Read the model definition and answer for the solid it produces. Units are mm, in the model's axes. Give positions to 0.01 mm unless a question says otherwise; leave off trailing zeros. Use a Markdown table: item, result.
from build123d import *

# Parameters (mm, degrees)
SKETCH1_W           = 79.799999912
SKETCH1_H           = 81.28
BOSS_EXTRUDE1_DEPTH = 1.600000102
SKETCH2_R           = 1.524
CUT_EXTRUDE1_DEPTH  = 107.841239355
SKETCH4_R           = 1.6
CUT_EXTRUDE2_DEPTH  = 107.841239355


with BuildPart() as part:
    # Sketch1 → Boss-Extrude1 (new body)
    with BuildSketch(Plane(origin=(0, 0, 0), x_dir=(1, 0, 0), z_dir=(0, 1, 0))):
        with Locations((-31.957523467, -38.410532915)):
            Rectangle(SKETCH1_W, SKETCH1_H)
    extrude(amount=BOSS_EXTRUDE1_DEPTH)

    # Sketch2 → Cut-Extrude1 (cut, through all)
    with BuildSketch(Plane(origin=(0, 1.600000102, 0), x_dir=(1, 0, 0), z_dir=(0, 1, 0))):
        with Locations(Location((5.842476489, -68.950532915, 0), (0, 0, 270))):
            Circle(SKETCH2_R)
    cut_extrude1 = extrude(amount=-CUT_EXTRUDE1_DEPTH, mode=Mode.SUBTRACT)

    # Mirror1: Cut-Extrude1 across plane
    add(cut_extrude1.mirror(Plane.XY.offset(38.410532915)), mode=Mode.SUBTRACT)

    # Sketch4 → Cut-Extrude2 (cut, through all)
    with BuildSketch(Plane.XZ):
        with Locations(Location((-67.657528223, 72.750532915, 0), (0, 0, 270))):
            Circle(SKETCH4_R)
    cut_extrude2 = extrude(amount=-CUT_EXTRUDE2_DEPTH, mode=Mode.SUBTRACT)

    # Mirror2: Cut-Extrude2 across plane
    add(cut_extrude2.mirror(Plane.XY.offset(38.410532915)), mode=Mode.SUBTRACT)


solid = part.part
Item 1: This flat-tipped pin is pushed along its axis until it touches: P1, Ø1.8, axis at x = 5.84, z = 68.95, coming from the +Y side. Where does it stop, or does it pass through?
Return value:
| item | result |
|---|---|
| P1 | through |
Item 2: Straight lines are drawn through the part: line 1 along X through (y, z) = (1.05, 69); line 2 along Z through (x, y) = (4.5, 0.2); line 3 along X through (y, z) = (0.6, 3). For each, find the intervals that lie inside material, in ascending order. Write a range as [from, to].
Return value:
| item | result |
|---|---|
| line 1 | [-71.86, 4.32], [7.37, 7.94] |
| line 2 | [-2.23, 7.15], [8.59, 68.23], [69.67, 79.05] |
| line 3 | [-71.86, -68.85], [-66.47, 7.94] |
Item 3: For a pull along X with two mould halves and no side action, classify faces 1 (the face through (-69.077, 0.789, 72.012)), 2 (the face through (-33, 1.6, 38)) as +X half, -X half, draft (parallel to the pull), parting line (faces both ways), or undercut.
Return value:
| item | result |
|---|---|
| face 1 | undercut |
| face 2 | draft |
